Model file for the job. Use its own axes, mm. A direction names the side the tool comes from. Coordinates: 2 decimals unless noted, no trailing zeros. Write each loop counter-clockwise with the first axis right and the second up, starting at its lowest first coordinate (ties: lowest second). Pieces come first, ordered by that corner, then holes.
Q1. Drill centre lines: probe 1 along Y at (x, z) = (-31, 2.45); probe 2 along Z at (x, y) = (-57.5, 5.5); probe 3 along Z at (x, y) = (-0.5, -3.25). Where is each one in solid material? Low to high.
Q2. Band-saw the part on A-A, the plane x = 15.5. Write the cut outline in (y, z), plus the area to 3 significant figures.
Q3. Pin check, flat tips, straight feed: P1, Ø1.5, axis at x = -17.5, y = -1, coming from the +Z side; P2, Ø4, axis at x = -31, y = 0.5, coming from the -Z side. Stop position of each tip, or through.
Q4. Band-saw the part on B-B, the plane z = 2.5. State how many separate pieces and enclosed holes the cut face has, plus the area to 3 significant figures.
Q5. Pull direction Y, two halves, no side cores. Call faces 1 (the flat face through (-1, 9, 3)), 2 (the flat face through (-2, 10.454, 1)), 3 (the flat face through (65, 1, 1)), 4 (the flat face through (-2, -9.546, 1)): released by +Y, released by -Y, zero draft, split by the parting line, or undercut.
Q6. Which spindle directions (+Z, -Z, +X, -X, +Y, -Y) get a long thin tool onto all of the face, cutting with end or side? Do faces 5 (the flat face through (-75.015, 0, 1)), 6 (the flat face through (-55, 1, 1)). Say none if no direction does.
from build123d import *

# Parameters (mm, degrees)
F0_W     = 148
F0_H     = 20
F1_DEPTH = 3
F2_W     = 10
F2_H     = 16
F3_DEPTH = 2
F4_R     = 2
F4_R_2   = 1.99999


# Not quite as in the source:
# - a fillet or chamfer is up to 0.001 mm smaller than in the source, because OpenCascade refuses the exact size


with BuildPart() as f1:
    # F0 (on Top) → F1 (new body)
    with BuildSketch(Plane.XY):
        with Locations((-1.0154450944, 0.4536062479)):
            Rectangle(F0_W, F0_H)
    extrude(amount=F1_DEPTH)

    # F2 (on face) → F3 (cut)
    with BuildSketch(Plane.XY.offset(3)):
        with Locations((-67.0154450944, 0.4536062479)):
            Rectangle(F2_W, F2_H)
        with Locations((-55.0154450944, 0.4536062479)):
            Rectangle(F2_W, F2_H)
        with Locations((-43.0154450944, 0.4536062479)):
            Rectangle(F2_W, F2_H)
        with Locations((-31.0154450944, 0.4536062479)):
            Rectangle(F2_W, F2_H)
        with Locations((-19.0154450944, 0.4536062479)):
            Rectangle(F2_W, F2_H)
        with Locations((-7.0154450944, 0.4536062479)):
            Rectangle(F2_W, F2_H)
        with Locations((4.9845549056, 0.4536062479)):
            Rectangle(F2_W, F2_H)
        with Locations((16.9845549056, 0.4536062479)):
            Rectangle(F2_W, F2_H)
        with Locations((28.9845549056, 0.4536062479)):
            Rectangle(F2_W, F2_H)
        with Locations((40.9845549056, 0.4536062479)):
            Rectangle(F2_W, F2_H)
        with Locations((52.9845549056, 0.4536062479)):
            Rectangle(F2_W, F2_H)
        with Locations((64.9845549056, 0.4536062479)):
            Rectangle(F2_W, F2_H)
    extrude(amount=-F3_DEPTH, mode=Mode.SUBTRACT)

    # F4 (call 1 of 16: OpenCascade refuses the feature's edges together)
    f4_edges = [f1.edges().sort_by_distance(p)[0] for p in [
        (-75.015445, -9.546394, 1.5),
    ]]
    fillet(f4_edges, radius=F4_R)

    # F4#2 (call 2 of 16)
    f4_2_edges = [f1.edges().sort_by_distance(p)[0] for p in [
        (72.984555, -9.546394, 1.5),
    ]]
    fillet(f4_2_edges, radius=F4_R)

    # F4#3 (call 3 of 16)
    f4_3_edges = [f1.edges().sort_by_distance(p)[0] for p in [
        (72.984555, 10.453606, 1.5),
    ]]
    fillet(f4_3_edges, radius=F4_R)

    # F4#4 (call 4 of 16)
    f4_4_edges = [f1.edges().sort_by_distance(p)[0] for p in [
        (-75.015445, 10.453606, 1.5),
    ]]
    fillet(f4_4_edges, radius=F4_R)

    # F4#5 (call 5 of 16) (radius 2 in the source; OpenCascade refuses exactly that, so slightly less here)
    f4_5_edges = [f1.edges().sort_by_distance(p)[0] for p in [
        (-72.015445, 0.453606, 3),
    ]]
    fillet(f4_5_edges, radius=F4_R_2)

    # F4#6 (call 6 of 16) (radius 2 in the source; OpenCascade refuses exactly that, so slightly less here)
    f4_6_edges = [f1.edges().sort_by_distance(p)[0] for p in [
        (-60.015445, 0.453606, 3),
    ]]
    fillet(f4_6_edges, radius=F4_R_2)

    # F4#7 (call 7 of 16) (radius 2 in the source; OpenCascade refuses exactly that, so slightly less here)
    f4_7_edges = [f1.edges().sort_by_distance(p)[0] for p in [
        (-48.015445, 0.453606, 3),
    ]]
    fillet(f4_7_edges, radius=F4_R_2)

    # F4#8 (call 8 of 16) (radius 2 in the source; OpenCascade refuses exactly that, so slightly less here)
    f4_8_edges = [f1.edges().sort_by_distance(p)[0] for p in [
        (-36.015445, 0.453606, 3),
    ]]
    fillet(f4_8_edges, radius=F4_R_2)

    # F4#9 (call 9 of 16) (radius 2 in the source; OpenCascade refuses exactly that, so slightly less here)
    f4_9_edges = [f1.edges().sort_by_distance(p)[0] for p in [
        (-24.015445, 0.453606, 3),
    ]]
    fillet(f4_9_edges, radius=F4_R_2)

    # F4#10 (call 10 of 16) (radius 2 in the source; OpenCascade refuses exactly that, so slightly less here)
    f4_10_edges = [f1.edges().sort_by_distance(p)[0] for p in [
        (-12.015445, 0.453606, 3),
    ]]
    fillet(f4_10_edges, radius=F4_R_2)

    # F4#11 (call 11 of 16) (radius 2 in the source; OpenCascade refuses exactly that, so slightly less here)
    f4_11_edges = [f1.edges().sort_by_distance(p)[0] for p in [
        (-0.015445, 0.453606, 3),
    ]]
    fillet(f4_11_edges, radius=F4_R_2)

    # F4#12 (call 12 of 16) (radius 2 in the source; OpenCascade refuses exactly that, so slightly less here)
    f4_12_edges = [f1.edges().sort_by_distance(p)[0] for p in [
        (11.984555, 0.453606, 3),
    ]]
    fillet(f4_12_edges, radius=F4_R_2)

    # F4#13 (call 13 of 16) (radius 2 in the source; OpenCascade refuses exactly that, so slightly less here)
    f4_13_edges = [f1.edges().sort_by_distance(p)[0] for p in [
        (23.984555, 0.453606, 3),
    ]]
    fillet(f4_13_edges, radius=F4_R_2)

    # F4#14 (call 14 of 16) (radius 2 in the source; OpenCascade refuses exactly that, so slightly less here)
    f4_14_edges = [f1.edges().sort_by_distance(p)[0] for p in [
        (35.984555, 0.453606, 3),
    ]]
    fillet(f4_14_edges, radius=F4_R_2)

    # F4#15 (call 15 of 16) (radius 2 in the source; OpenCascade refuses exactly that, so slightly less here)
    f4_15_edges = [f1.edges().sort_by_distance(p)[0] for p in [
        (47.984555, 0.453606, 3),
    ]]
    fillet(f4_15_edges, radius=F4_R_2)

    # F4#16 (call 16 of 16) (radius 2 in the source; OpenCascade refuses exactly that, so slightly less here)
    f4_16_edges = [f1.edges().sort_by_distance(p)[0] for p in [
        (59.984555, 0.453606, 3),
    ]]
    fillet(f4_16_edges, radius=F4_R_2)


solid = f1.part
Answer sheet:
1. probe 1: y = -9.55 to -7.55, 8.45 to 10.45
1. probe 2: z = 0 to 1
1. probe 3: z = 0 to 2.31
2. outline: (-9.55, 0) - (10.45, 0) - (10.45, 3) - (8.45, 3) - (8.45, 1) - (-7.55, 1) - (-7.55, 3) - (-9.55, 3) - close
2. area: 28.0 mm2
3. P1: stops at z = 1
3. P2: stops at z = 0
4. separate pieces: 1
4. enclosed holes: 12
4. area: 907 mm2
5. face 1: zero draft
5. face 2: released by +Y
5. face 3: undercut
5. face 4: released by -Y
6. face 5: +Z, -Z, -X, +Y, -Y
6. face 6: +Z
